Model file for the job. Use its own axes, mm. Face numbers are marked on the shaded views. A direction names the side the tool comes from. Coordinates: 2 decimals unless noted, no trailing zeros. Loops run counter-clockwise (first coordinate to the right, second up) from the corner with the lowest first, then second, coordinate; pieces in that order, holes last.
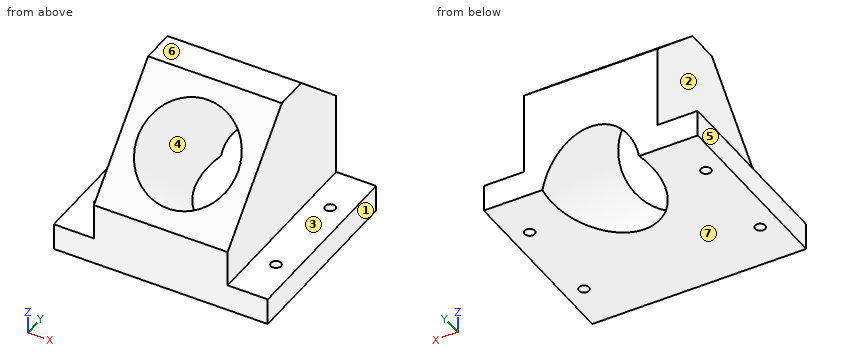
from build123d import *

# Parameters (mm, degrees)
F0_W     = 280
F0_H     = 40
F1_DEPTH = 160
F2_DEPTH = 100
F3_R     = 7.5
F4_DEPTH = 50
F5_R     = 75
F6_DEPTH = 421.5


with BuildPart() as f1:
    # F0 (on Right) → F1 (new body, symmetric)
    with BuildSketch(Plane.YZ):
        with Locations((0, -12.4763777256)):
            Rectangle(F0_W, F0_H)
    extrude(amount=F1_DEPTH, both=True)

    # F0 (on Right) → F2 (join, symmetric)
    with BuildSketch(Plane.YZ):
        Polygon((-140, 61.5236222744), (-140, 7.5236222744), (140, 7.5236222744), (140, 131.5236222744), (50, 211.5236222744), (0, 211.5236222744), align=None)
    extrude(amount=F2_DEPTH, both=True)

    # F3 (on face) → F4 (cut)
    with BuildSketch(Plane.XY.offset(7.5236222744)):
        with Locations((-131.7980587482, 70)):
            Circle(F3_R)
        with Locations((-131.7980587482, -70)):
            Circle(F3_R)
        with Locations((131.7980587482, 70)):
            Circle(F3_R)
        with Locations((131.7980587482, -70)):
            Circle(F3_R)
    extrude(amount=-F4_DEPTH, mode=Mode.SUBTRACT)

    # F5 (on face) → F6 (cut)
    with BuildSketch(Plane(origin=(0, -105.5105954338, 98.4765557382), x_dir=(1, 0, 0), z_dir=(0, -0.7310552682, 0.6823182504))):
        with Locations((0, 52.0439584215)):
            Circle(F5_R)
    extrude(amount=-F6_DEPTH, mode=Mode.SUBTRACT)


solid = f1.part
Q1. Slice it at A-A (x = -24.5). List the corners of the cut face in (y, z), and give its area (3 significant figures).
Answers:
outline: (-140, -32.48) - (7.18, -32.48) - (-118.37, 84.7) - (-140, 61.52) - close; (-21.63, 188.34) - (140, 37.49) - (140, 131.52) - (50, 211.52) - (0, 211.52) - close
area: 21,700 mm2
Q2. Drill centre lines: line 1 (X direction, y = -69, z = 1); line 2 (Z direction, x = -101, y = 126.5); line 3 (X direction, y = 129, z = 17). Where is each one in solid material? Low to high.
Answers:
line 1: x = -160 to -139.23, -124.37 to 124.37, 139.23 to 160
line 2: z = -32.48 to 7.52
line 3: x = -100 to -57.29, 57.29 to 100
Q3. Which spindle directions (+Z, -Z, +X, -X, +Y, -Y) get a long thin tool onto all of the face, cutting with end or side? Do the marked faces 1, 2 and 3. Say none if no direction does.
Answers:
face 1: +Z, -Z, +X, +Y, -Y
face 2: +Z, -X, +Y, -Y
face 3: +Z, +X, +Y, -Y
Q4. Flat gauge pins, fed straight in: P1, Ø10, axis at x = 11.5, y = -8.5, coming from the +Z side; P2, Ø17, axis at x = -131.8, y = -70, coming from the +Z side; P3, Ø2, axis at y = 110, z = 78, coming from the +X side. Where does each tip first touch, or does it go through?
Answers:
P1: stops at z = 207.77
P2: stops at z = 7.52
P3: stops at x = 100
Q5. Slice it at B-B (y = 70). Count the separate pieces of the cut face and the enclosed holes in it, and give its area (3 significant figures).
Answers:
separate pieces: 3
enclosed holes: 0
area: 31,100 mm2
Q6. Mould opens along Z. For the marked faces 4, 5, 6 and 7 say: +Z half, -Z half, draft (parallel to the pull), parting line (faces both ways), or undercut.
Answers:
face 4: undercut
face 5: draft
face 6: +Z half
face 7: -Z half
